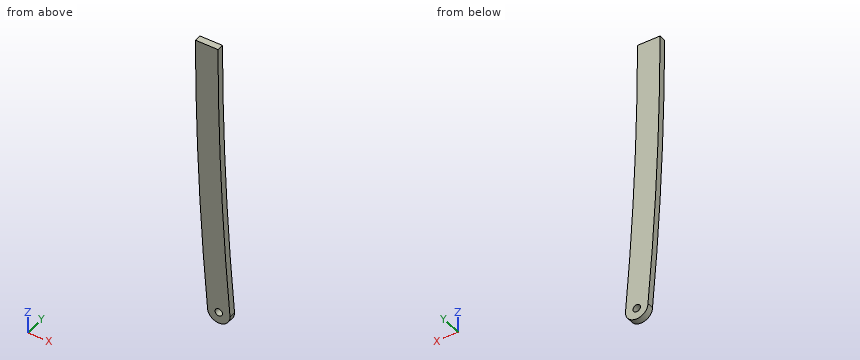
Autodesk Inventor part; units mm, degrees
ref_plane "YZ Plane" through (0, 0, 0) normal (1, 0, 0) x (0, 1, 0)
ref_plane "XZ Plane" through (0, 0, 0) normal (0, 1, 0) x (-1, 0, 0)
ref_plane "XY Plane" through (0, 0, 0) normal (0, 0, 1) x (1, 0, 0)
sketch "Sketch1" plane through (0, 0, 0) normal (0, 1, 0) x (-1, 0, 0)
  line L0 (0, 0) -> (0, -253.429) construction
  line L1 (5, 0) -> (5, -253.429)
  line L2 (-5, -253.429) -> (-5, 0)
  arc A0 (5, 0) -> (-5, 0) centre (0, 0) ccw
  arc A1 (-5, -253.429) -> (5, -253.429) centre (0, -253.429) ccw
  circle A2 centre (0, 0) radius 1.65
  circle A3 centre (0, -253.429) radius 1.65
  arc A4 (5, -253.429) -> (5, 0) centre (-1489.6382, -126.7145) ccw
  arc A5 (-5, -253.429) -> (-5, 0) centre (-1499.6382, -126.7145) ccw
  point P0 (0, -126.7145)
  dimension "d0" = 3.3
  dimension "d1" = 3.3
  dimension "d2" = 10
  dimension "d3" = 253.429
  dimension "d16" = 1500
  dimension "d17" = 1500
extrude "Extrusion1" add sketch "Sketch1" along normal blind 3 contours A4 L1 | L1 A1 A5 A0
sketch "Sketch2" plane through (0, 3, 0) normal (0, 1, 0) x (1, 0, 0)
  line L0 (-27.9396, 271.9091) -> (26.8888, 271.9091)
  line L1 (26.8888, 271.9091) -> (26.8888, 130.022)
  line L2 (26.8888, 130.022) -> (-27.9396, 130.022)
  line L3 (-27.9396, 130.022) -> (-27.9396, 271.9091)
  line L4 (-79.0634, 296.7301) -> (75.0489, 296.7301)
  line L5 (75.0489, 296.7301) -> (75.0489, -47.4295)
  line L6 (75.0489, -47.4295) -> (-79.0634, -47.4295)
  line L7 (-79.0634, -47.4295) -> (-79.0634, 296.7301)
  point P0 (0, 0)
extrude "Extrusion2" cut sketch "Sketch2" against normal blind 10
properties part number "Part_8_p2"
Geometry: final body of the model. Coordinates: model frame, mm. Coordinates: 2 decimals unless noted, no trailing zeros. Order: outer loops, then holes, each group sorted by start corner. A loop starts at its lowest first (then second) coordinate and runs counter-clockwise, first axis right, second up. Notation, with made-up numbers: M 41,-38 L 76,-38 A27 cw 76,-11 Z; hole C -6,7.25 d2. An arc over 180 degrees is marked long. Answer as CSV lines item,"result".
Q1. Section B-B on z = -169. Return the cut outline in (x, y), and give its area (3 significant figures).
Answers:
outline,"M -9.77,0 L 0.23,0 L 0.23,3 L -9.77,3 Z"
area,"30.0 mm^2"
Q2. First-contact query: P1, Ø4.5, axis at x = 0, z = -253.429, coming from the -Y side; P2, Ø1, axis at x = -1.5, y = 2, coming from the -Z side. Flat tips, straight axial feed; report the tip coordinate or a pass-through.
Answers:
P1,"stops at y = 0"
P2,"stops at z = -258.33"
Q3. Line query: probe 1 along X at (y, z) = (2.2, -204.5); probe 2 along X at (y, z) = (2.05, -226); probe 3 along Z at (x, y) = (-4, 1.15). Output: solid intervals per line, ascending. Write a range as [from, to].
Answers:
probe 1,"x = [-8.34, 1.66]"
probe 2,"x = [-7.07, 2.93]"
probe 3,"z = [-256.43, -130.02]"
Q4. Section A-A on y = 0.85. Return the cut outline in (x, z), and give its area (3 significant figures).
Answers:
outline,"M -10.36,-130.02 A1500 ccw -5,-253.43 A5 ccw 5,-253.43 A1500 cw -0.36,-130.02 Z; hole C 0,-253.43 d3.3"
area,"1,260 mm^2"
